Can you work these out from the model? Positions are in its coordinate system, mm. A direction names the side the tool comes from. Give positions to 0.01 mm unless a question says otherwise; leave off trailing zeros. Order: outer loops, then holes, each group sorted by start corner. A loop starts at its lowest first (then second) coordinate and runs counter-clockwise, first axis right, second up. Notation, with made-up numbers: M 75.25,85 L 100.25,85 A15 cw 100.25,109 Z; hole C 13.25,85 d8. An arc over 180 degrees is marked long. One line per question, with ' | ' between items. Start each with the question number.
1) If we section it at A-A, the plane z = 12: Please give me the cut outline in (x, y), plus the area to 3 significant figures.
2) For faces 4 (the flat face through (-12, 1, 31.402)), 5 (the flat face through (-90.3, 1, 19)), 6 (the flat face through (-49, 1, 5.752)), which set-ups out of +Z, -Z, +X, -X, +Y, -Y let a thin tool reach every point of the face, with its end or its side?
3) I'm going to push flat-ended pins straight in: pin 1 Ø0.8 at (x, y) = (-60.5, 0.5) entering from +Z; pin 2 Ø0.7 at (x, y) = (-95.5, 0.5) entering from +Z; pin 3 Ø4 at (x, z) = (-35.5, 6) entering from -Y; pin 4 Ø0.8 at (y, z) = (1, 16.5) entering from -X. Where does each tip first touch, or does it pass through?
4) Please list where these lines run through material, in increasing order: line 1 along X through (y, z) = (1, 0); line 2 along X through (y, z) = (0.85, 22); line 3 along Z through (x, y) = (0, 0.4). Write a range as [from, to].
5) If we section it at B-B, the plane z = 0: Please give me the cut outline in (x, y), plus the area to 3 significant figures.
6) Thinking about a two-plate mould opening in X: for faces 1 (the flat face through (-4.7, 1, 19)), 2 (the cylindrical face through (-91.64, 0.789, 5.213)), 3 (the flat face through (-17.75, 1, 19)), which applies, +X half, -X half, draft (parallel to the pull), parting line (faces both ways), or undercut?
```python
from build123d import *

# Parameters (mm, degrees)
SKETCH1_R           = 1.5
BOSS_EXTRUDE1_DEPTH = 1.6
FILLET1_R           = 1


with BuildPart() as part:
    # Sketch1 → Boss-Extrude1 (new body)
    with BuildSketch(Plane(origin=(0, 0, 0), x_dir=(1, 0, 0), z_dir=(0, 1, 0))):
        with BuildLine():
            Line((0.9, -3.8), (0, -3.8))
            ThreePointArc((0, -3.8), (-3.323401872, -5.176598128), (-4.7, -8.5))
            Line((-4.7, -8.5), (-4.7, -28.901853444))
            ThreePointArc((-4.7, -28.901853444), (-5.432233047, -30.669620397), (-7.2, -31.401853444))
            Line((-7.2, -31.401853444), (-17.75, -31.401853444))
            Line((-17.75, -31.401853444), (-17.75, -5.751853444))
            Line((-17.75, -5.751853444), (-81.45, -5.751853444))
            Line((-81.45, -5.751853444), (-81.45, -31.401853444))
            Line((-81.45, -31.401853444), (-87.8, -31.401853444))
            ThreePointArc((-87.8, -31.401853444), (-89.567766953, -30.669620397), (-90.3, -28.901853444))
            Line((-90.3, -28.901853444), (-90.3, -8.5))
            ThreePointArc((-90.3, -8.5), (-91.676598128, -5.176598128), (-95, -3.8))
            Line((-95, -3.8), (-95.9, -3.8))
            ThreePointArc((-95.9, -3.8), (-96.960660172, -3.360660172), (-97.4, -2.3))
            Line((-97.4, -2.3), (-97.4, 2.67635027))
            ThreePointArc((-97.4, 2.67635027), (-96.976459398, 3.720972291), (-95.94501978, 4.175674525))
            add(Edge.make_bspline(
                [(0.94501978, 4.175674525), (-47.5, 5.630319254), (-95.94501978, 4.175674525)],
                knots=[4.549425728, 4.549425728, 4.549425728, 4.875352233, 4.875352233, 4.875352233], degree=2, weights=[1, 0.98675085, 1]))
            ThreePointArc((0.94501978, 4.175674525), (1.976459398, 3.720972291), (2.4, 2.67635027))
            Line((2.4, 2.67635027), (2.4, -2.3))
            ThreePointArc((2.4, -2.3), (1.960660172, -3.360660172), (0.9, -3.8))
        make_face()
        Circle(SKETCH1_R, mode=Mode.SUBTRACT)
    extrude(amount=BOSS_EXTRUDE1_DEPTH)

    # Fillet1
    fillet1_edges = [part.edges().sort_by_distance(p)[0] for p in [
        (-17.75, 0.8, 5.751853444),
        (-81.45, 0.8, 5.751853444),
    ]]
    fillet(fillet1_edges, radius=FILLET1_R)


solid = part.part
```
Results found:
1) outline: M -90.3,0 L -81.45,0 L -81.45,1.6 L -90.3,1.6 Z; M -17.75,0 L -4.7,0 L -4.7,1.6 L -17.75,1.6 Z | area: 35.0 mm²
2) face 4: +Z, +X, -X, +Y, -Y | face 5: +Z, -X, +Y, -Y | face 6: +Z, +Y, -Y
3) pin 1: stops at z = 5.75 | pin 2: stops at z = 3.8 | pin 3: stops at y = 0 | pin 4: stops at x = -90.3
4) line 1: x = [-97.4, -1.5], [1.5, 2.4] | line 2: x = [-90.3, -81.45], [-17.75, -4.7] | line 3: z = [-4.2, -1.5], [1.5, 3.8]
5) outline: M -97.4,0 L -1.5,0 L -1.5,1.6 L -97.4,1.6 Z; M 1.5,0 L 2.4,0 L 2.4,1.6 L 1.5,1.6 Z | area: 155 mm²
6) face 1: +X half | face 2: -X half | face 3: undercut
